Autodesk Inventor part; units mm, degrees
ref_plane "YZ Plane" through (0, 0, 0) normal (1, 0, 0) x (0, 1, 0)
ref_plane "XZ Plane" through (0, 0, 0) normal (0, 1, 0) x (-1, 0, 0)
ref_plane "XY Plane" through (0, 0, 0) normal (0, 0, 1) x (1, 0, 0)
sketch "Sketch1" plane through (0, 0, 0) normal (0, 0, 1) x (1, 0, 0)
  circle A0 centre (0, 0) radius 15.24
  circle A1 centre (0, -7.62) radius 5.08
  dimension "d0" = 30.48
  dimension "d1" = 10.16
  dimension "d2" = 7.62
extrude "Extrusion1" add sketch "Sketch1" against normal blind 58.42 contours A0 | A1
extrude "Extrusion2" add sketch "Sketch1" along normal blind 25.4 contours A1
sketch "Sketch2" plane through (0, 0, 0) normal (1, 0, 0) x (0, 1, 0)
  line L0 (15.24, 0) -> (15.24, -58.42)
  line L1 (15.24, -58.42) -> (-15.24, -58.42)
  line L2 (-15.24, -58.42) -> (-15.24, 0)
  line L3 (-15.24, 0) -> (-12.7, 0)
  line L4 (-12.7, 0) -> (-12.7, 25.4)
  line L5 (-12.7, 25.4) -> (-2.54, 25.4)
  line L6 (-2.54, 25.4) -> (-2.54, 0)
  line L7 (-2.54, 0) -> (15.24, 0)
  line L8 (-15.24, -58.42) -> (15.24, -58.42)
  line L9 (15.24, 0) -> (-15.24, 0)
  circle A0 centre (0, -45.72) radius 3.81
  point P0 (0, 0)
  dimension "d7" = 7.62
  dimension "d8" = 12.7
extrude "Extrusion3" cut sketch "Sketch2" against normal through all both and the other way through all contours A0
chamfer "Chamfer1" distance 0.635 angle 45 1 edges at (-5.08, -7.62, 25.4) measured on face at (5.0635, -8.0288, 16.9333)
chamfer "Chamfer2" distance 1.27 angle 45 2 edges at (-15.24, 0, -58.42) (-15.24, 0, 0) measured on face at (9.6385, 11.805, -38.9467)
equation "\"BendRadius\" = Thickness"
equation "\"BendReliefWidth\" = Thickness"
equation "\"BendReliefDepth\" = 0.5 * Thickness"
equation "\"CornerReliefSize\" = 4 * Thickness"
equation "\"MinimumRemnant\" = 2 * Thickness"
equation "\"TransitionRadius\" = BendRadius"
equation "\"JacobiRadiusSize\" = BendRadius"
equation "\"GapSize\" = Thickness"
properties part number "crankshaft valve crank" material "Stainless Steel"
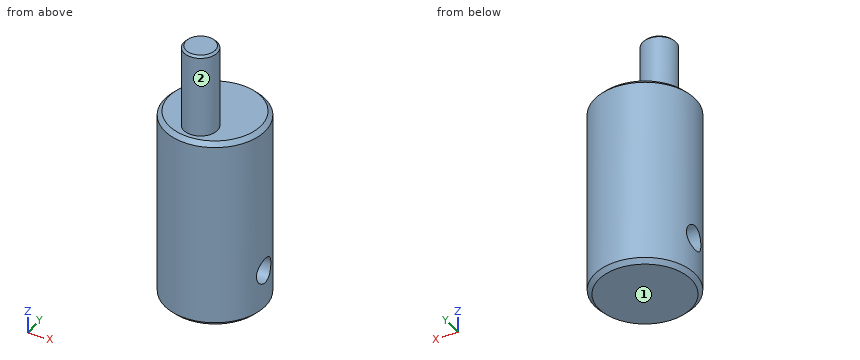
CAD build for the part. Positions are in the model's coordinates, mm. Face numbers are marked on the shaded views. A direction names the side the tool comes from. Round coordinates to 2 decimals unless told otherwise and drop trailing zeros. Loops run counter-clockwise (first coordinate to the right, second up) from the corner with the lowest first, then second, coordinate; pieces in that order, holes last. Notation, with made-up numbers: (74, 44) - (124, 44) arc R18 ccw to (124, 72) - close; hole circle Ø2 at (58, 10). An arc over 180 degrees is marked (long way). Return JSON: item names as keys, results as strings. Group by question number.
Q1. Band-saw the part on D-D on z = -7. Give the cut face in (x, y).
Q2. Drill centre lines: line 1 along Z through (x, y) = (6, 0); line 2 along Z through (x, y) = (-2, 3.5); line 3 along Z through (x, y) = (4, 12.5). Where is each one in solid material? Low to high. Write a range as [from, to].
Q3. Tool access for the marked faces 1 and 2: list every direction of +Z, -Z, +X, -X, +Y, -Y with a clear straight run to the whole face (end or side of a thin tool).
Q4. Band-saw the part on C-C on z = -45.72. Give the cut face in (x, y), plus the area to 3 significant figures.
Q5. Band-saw the part on A-A on x = 0. Give the cut face in (y, z) (3 decimals).
Q6. Band-saw the part on B-B on y = 0. Give the cut face in (x, z), plus the area to 3 significant figures.
Q7. Flat gauge pins, fed straight in: pin 1 Ø4 at (x, z) = (-9.5, -12) entering from -Y; pin 2 Ø1 at (x, z) = (-6, -45) entering from +Y; pin 3 Ø12 at (x, y) = (-10, 2.5) entering from +Z. Where does each tip first touch, or does it go through?
Solutions:
{
 "1": {"outline": "circle Ø30.48 at (0, 0)"},
 "2": {"line 1": "z = [-58.42, -49.53], [-41.91, 0]", "line 2": "z = [-58.42, -47.23], [-44.21, 0]", "line 3": "z = [-58.42, 0]"},
 "3": {"face 1": "-Z, +X, -X, +Y, -Y", "face 2": "+Z"},
 "4": {"outline": "(-14.76, -3.81) arc R15.24 ccw to (14.76, -3.81) - close; (-14.76, 3.81) - (14.76, 3.81) arc R15.24 ccw to start", "area": "500 mm^2"},
 "5": {"outline": "(-15.24, -57.15) - (-13.97, -58.42) - (13.97, -58.42) - (15.24, -57.15) - (15.24, -1.27) - (13.97, 0) - (-2.54, 0) - (-2.54, 24.765) - (-3.175, 25.4) - (-12.065, 25.4) - (-12.7, 24.765) - (-12.7, 0) - (-13.97, 0) - (-15.24, -1.27) - close; hole circle Ø7.62 at (0, -45.72)"},
 "6": {"outline": "(-15.24, -57.15) - (-13.97, -58.42) - (13.97, -58.42) - (15.24, -57.15) - (15.24, -49.53) - (-15.24, -49.53) - close; (-15.24, -41.91) - (15.24, -41.91) - (15.24, -1.27) - (13.97, 0) - (-13.97, 0) - (-15.24, -1.27) - close", "area": "1,550 mm^2"},
 "7": {"pin 1": "stops at y = -13.27", "pin 2": "stops at y = 14.21", "pin 3": "stops at z = 0"}
}
